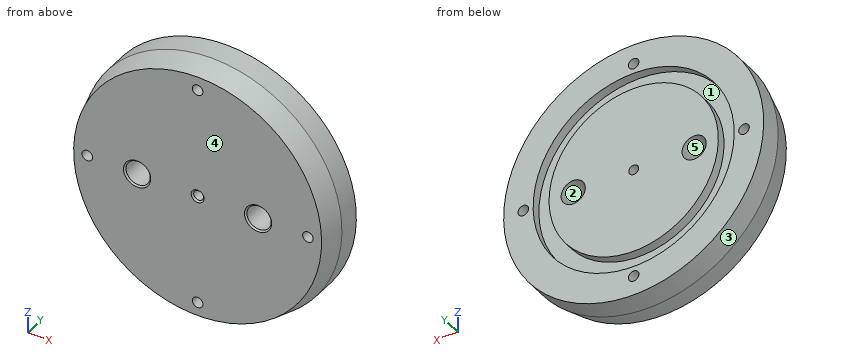
```python
from build123d import *

# Parameters (mm, degrees)
SKETCH1_R           = 43
BOSS_EXTRUDE1_DEPTH = 15
SKETCH2_R           = 4
CUT_EXTRUDE1_DEPTH  = 63.633856659
SKETCH3_R           = 1.625
CUT_EXTRUDE2_DEPTH  = 63.633856659
SKETCH4_R           = 33.25
SKETCH4_R_2         = 28
CUT_EXTRUDE3_DEPTH  = 3
SKETCH5_R           = 1.75
CUT_EXTRUDE4_DEPTH  = 63.633856659
CIRPATTERN1_COUNT   = 4
CHAMFER1_SIZE       = 2
CHAMFER1_SIZE2      = 7.464101615
CHAMFER2_SIZE       = 0.5


with BuildPart() as part:
    # Sketch1 → Boss-Extrude1 (new body)
    with BuildSketch(Plane(origin=(0, 0, 0), x_dir=(1, 0, 0), z_dir=(0, 1, 0))):
        with Locations(Location((0, 0, 0), (0, 0, 270))):
            Circle(SKETCH1_R)
    extrude(amount=BOSS_EXTRUDE1_DEPTH)

    # Sketch2 → Cut-Extrude1 (cut, through all)
    with BuildSketch(Plane.XZ):
        with Locations(Location((20, 0, 0), (0, 0, 270))):
            Circle(SKETCH2_R)
        with Locations(Location((-20, 0, 0), (0, 0, 270))):
            Circle(SKETCH2_R)
    extrude(amount=-CUT_EXTRUDE1_DEPTH, mode=Mode.SUBTRACT)

    # Sketch3 → Cut-Extrude2 (cut, through all)
    with BuildSketch(Plane(origin=(0, 15, 0), x_dir=(1, 0, 0), z_dir=(0, 1, 0))):
        with Locations(Location((0, 0, 0), (0, 0, 270))):
            Circle(SKETCH3_R)
    extrude(amount=-CUT_EXTRUDE2_DEPTH, mode=Mode.SUBTRACT)

    # Sketch4 → Cut-Extrude3 (cut)
    with BuildSketch(Plane(origin=(0, 15, 0), x_dir=(1, 0, 0), z_dir=(0, 1, 0))):
        with Locations(Location((0, 0, 0), (0, 0, 270))):
            Circle(SKETCH4_R)
        with Locations(Location((0, 0, 0), (0, 0, 270))):
            Circle(SKETCH4_R_2, mode=Mode.SUBTRACT)
    extrude(amount=-CUT_EXTRUDE3_DEPTH, mode=Mode.SUBTRACT)

    # Sketch5 → Cut-Extrude4 (cut, through all)
    with BuildSketch(Plane.XZ):
        with Locations(Location((36.5, 0, 0), (0, 0, 270))):
            Circle(SKETCH5_R)
    cut_extrude4 = extrude(amount=-CUT_EXTRUDE4_DEPTH, mode=Mode.SUBTRACT)

    # CirPattern1: Cut-Extrude4 ×4 about axis
    cirpattern1_axis = Axis((0, 0, 0), (0, 1, 0))
    for i in range(1, CIRPATTERN1_COUNT):
        add(cut_extrude4.rotate(cirpattern1_axis, i * 360 / CIRPATTERN1_COUNT), mode=Mode.SUBTRACT)

    # Chamfer1
    chamfer1_edges = [part.edges().sort_by_distance(p)[0] for p in [
        (0, 0, -43),
    ]]
    chamfer1_side = [part.faces().sort_by_distance(p)[0] for p in [
        (0, 0, -41.783776336),
    ]]
    chamfer(chamfer1_edges, length=CHAMFER1_SIZE, length2=CHAMFER1_SIZE2, reference=chamfer1_side[0])

    # Chamfer2
    chamfer2_edges = [part.edges().sort_by_distance(p)[0] for p in [
        (-20, 0, 4),
        (0, 0, -1.625),
        (20, 0, 4),
    ]]
    chamfer(chamfer2_edges, length=CHAMFER2_SIZE)


solid = part.part
```
Verification items for the finished model (mm, model axes). Face numbers are marked on the shaded views. A direction names the side the tool comes from. Round coordinates to 2 decimals unless told otherwise and drop trailing zeros. Write each loop counter-clockwise with the first axis right and the second up, starting at its lowest first coordinate (ties: lowest second). Pieces come first, ordered by that corner, then holes.
1. Scan lines: L1, parallel to X at y = 8.25, z = 0 (3 decimals); L2, parallel to X at y = 13.75, z = -12.5; L3, parallel to X at y = 7, z = -1. Record each from-to range of solid material in increasing order.
2. Access from +Z, -Z, +X, -X, +Y, -Y to the whole of each face (thin tool, end or side, straight path). Record for the marked faces 1 and 2.
3. Section check B-B on z = 0. State how many separate pieces and enclosed holes the cut face has, plus the area to 3 significant figures.
4. Section check A-A on x = 0. Enter the section's corners in (y, z) (3 decimals).
5. Gauge pin test, flat ends, axial feed: P1, Ø8, axis at y = 13, z = -1, coming from the -X side; P2, Ø5, axis at x = -16.5, y = 13.5, coming from the +Z side; P3, Ø8, axis at x = -7, y = 2.5, coming from the +Z side; P4, Ø13, axis at x = -20, z = 0, coming from the +Y side. Record the tip position at first contact, or that the pin passes through.
6. Draft check along Z on the marked faces 3, 4 and 5. Enter one of: +Z half, -Z half, draft (parallel to the pull), parting line (faces both ways), or undercut.
Answer:
1. L1: x = -43 to -38.25, -34.75 to -24, -16 to -1.625, 1.625 to 16, 24 to 34.75, 38.25 to 43
1. L2: x = -41.14 to -30.81, -25.05 to 25.05, 30.81 to 41.14
1. L3: x = -42.86 to -37.94, -35.06 to -23.87, -16.13 to -1.28, 1.28 to 16.13, 23.87 to 35.06, 37.94 to 42.86
2. face 1: +Y
2. face 2: +Y, -Y
3. separate pieces: 6
3. enclosed holes: 0
3. area: 849 mm2
4. outline: (0, -41) - (7.464, -43) - (15, -43) - (15, -38.25) - (0, -38.25) - close; (0, -34.75) - (15, -34.75) - (15, -33.25) - (12, -33.25) - (12, -28) - (15, -28) - (15, -1.625) - (0.5, -1.625) - (0, -2.125) - close; (0, 2.125) - (0.5, 1.625) - (15, 1.625) - (15, 28) - (12, 28) - (12, 33.25) - (15, 33.25) - (15, 34.75) - (0, 34.75) - close; (0, 38.25) - (15, 38.25) - (15, 43) - (7.464, 43) - (0, 41) - close
5. P1: stops at x = -43
5. P2: stops at z = 40.66
5. P3: stops at z = 42.31
5. P4: stops at y = 15
6. face 3: parting line
6. face 4: draft
6. face 5: undercut
